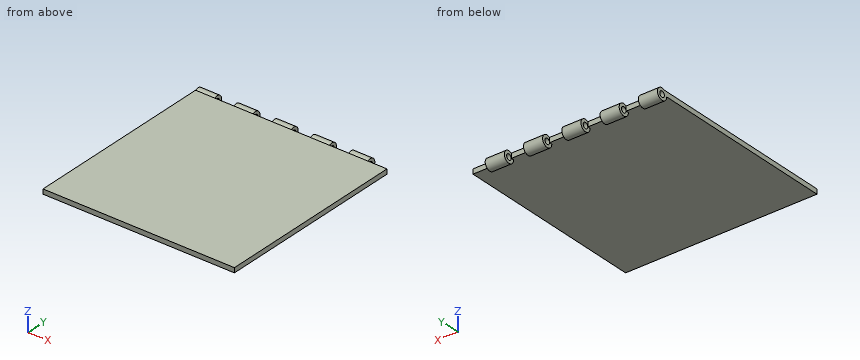
from build123d import *

# Parameters (mm, degrees)
SKETCH1_W           = 254
SKETCH1_H           = 254
BOSS_EXTRUDE1_DEPTH = 3.175
SKETCH2_R           = 7.62
SKETCH2_R_2         = 3.81
BOSS_EXTRUDE2_DEPTH = 25.4
LPATTERN1_COUNT     = 5
LPATTERN1_PITCH     = 50.8
SCALE1_SCALE        = 0.9


with BuildPart() as part:
    # Sketch1 → Boss-Extrude1 (new, symmetric)
    with BuildSketch(Plane.XY):
        with Locations((127, 127)):
            Rectangle(SKETCH1_W, SKETCH1_H)
    extrude(amount=BOSS_EXTRUDE1_DEPTH, both=True)

    # Sketch2 → Boss-Extrude2 (add)
    with BuildSketch(Plane.ZY):
        with Locations((-3.35543862, 257.92654701)):
            Circle(SKETCH2_R)
        with Locations(Location((-3.35543862, 257.92654701, 0), (0, 0, 270))):
            Circle(SKETCH2_R_2, mode=Mode.SUBTRACT)
    boss_extrude2 = extrude(amount=-BOSS_EXTRUDE2_DEPTH)

    # LPattern1: Boss-Extrude2 ×5
    with Locations(*[(i * LPATTERN1_PITCH, 0, 0) for i in range(1, LPATTERN1_COUNT)]):
        add(boss_extrude2)


with BuildPart() as part_1:
    # Scale1: scaled about (126.542998423, 131.737903525, -0.133748204)
    add(part.part.scale(SCALE1_SCALE).moved(Location((12.654299842, 13.173790352, -0.01337482))))


solid = part_1.part
Read the model definition and answer for the solid it produces. Units are mm, in the model's axes. Coordinates: 2 decimals unless noted, no trailing zeros. Loops run counter-clockwise (first coordinate to the right, second up) from the corner with the lowest first, then second, coordinate; pieces in that order, holes last. Notation, with made-up numbers: (60.5, -20.5) -> (65.5, -20.5) arc R19 cw to (65.5, -16.5) -> close; hole circle Ø1 at (20.25, 72). An arc over 180 degrees is marked (long way). Write item = value, one per line. Start each with the question number.
1) The part is cut by section B-B, the plane x = 162.5. Determine the outline of the cut face in (y, z).
2) Find the intervals of material crossed by L1, parallel to Y at x = 54.5, z = -0.75; L2, parallel to Z at x = 175.5, y = 150; L3, parallel to Y at x = 111.5, z = -1, in increasing order. Write a range as from..to.
3) Given P1, Ø6, axis at x = 211.5, y = 137.5, coming from the -Z side; P2, Ø5.5, axis at y = 245.31, z = -3.03, coming from the +X side (3 decimals); P3, Ø6.5, axis at x = 43.5, z = 0, coming from the +Y side; P4, Ø4, axis at x = 103.5, z = 1, coming from the +Y side, each flat-ended and moving along its own axis, determine where each tip first touches the part or whether it passes through.
4) The part is cut by section A-A, the plane y = 74. Determine the outline of the cut face in (x, z).
5) The part is cut by section C-C, the plane x = 94. Determine the outline of the cut face in (y, z).
Result:
q1.outline = (13.17, -2.87) -> (238.45, -2.87) arc R6.86 ccw (long way) to (241.77, 2.84) -> (13.17, 2.84) -> close; hole circle Ø6.86 at (245.31, -3.03)
q2.L1 = 13.17..241.77
q2.L2 = -2.87..2.84
q2.L3 = 13.17..242.55, 248.07..251.86
q3.P1 = -2.87
q3.P2 = through
q3.P3 = 241.77
q3.P4 = 251.83
q4.outline = (12.65, -2.87) -> (241.25, -2.87) -> (241.25, 2.84) -> (12.65, 2.84) -> close
q5.outline = (13.17, -2.87) -> (241.77, -2.87) -> (241.77, 2.84) -> (13.17, 2.84) -> close
